Autodesk Inventor part; units mm, degrees
ref_plane "YZ Plane" through (0, 0, 0) normal (1, 0, 0) x (0, 1, 0)
ref_plane "XZ Plane" through (0, 0, 0) normal (0, 1, 0) x (-1, 0, 0)
ref_plane "XY Plane" through (0, 0, 0) normal (0, 0, 1) x (1, 0, 0)
sketch "Sketch1" plane through (0, 0, 0) normal (0, 1, 0) x (-1, 0, 0)
  circle A0 centre (0, 0) radius 13
  line L0 (-11.5, 0) -> (-9.303695, 6.75953) construction
  line L1 (-9.303695, 6.75953) -> (-3.553695, 10.93715) construction
  line L2 (-3.553695, 10.93715) -> (3.553695, 10.93715) construction
  line L3 (3.553695, 10.93715) -> (9.303695, 6.75953) construction
  line L4 (9.303695, 6.75953) -> (11.5, 0) construction
  line L5 (11.5, 0) -> (9.303695, -6.75953) construction
  line L6 (9.303695, -6.75953) -> (3.553695, -10.93715) construction
  line L7 (3.553695, -10.93715) -> (-3.553695, -10.93715) construction
  line L8 (-3.553695, -10.93715) -> (-9.303695, -6.75953) construction
  line L9 (-9.303695, -6.75953) -> (-11.5, 0) construction
  circle A1 centre (-6, 0) radius 3 construction
  circle A2 centre (6, 0) radius 3 construction
  line L10 (13, 0) -> (10.517221, -7.641208) construction
  line L11 (10.517221, -7.641208) -> (4.017221, -12.363735) construction
  line L12 (4.017221, -12.363735) -> (-4.017221, -12.363735) construction
  line L13 (-4.017221, -12.363735) -> (-10.517221, -7.641208) construction
  line L14 (-10.517221, -7.641208) -> (-13, 0) construction
  line L15 (-13, 0) -> (-10.517221, 7.641208) construction
  line L16 (-10.517221, 7.641208) -> (-4.017221, 12.363735) construction
  line L17 (-4.017221, 12.363735) -> (4.017221, 12.363735) construction
  line L18 (4.017221, 12.363735) -> (10.517221, 7.641208) construction
  line L19 (10.517221, 7.641208) -> (13, 0) construction
  dimension "d0" = 26
  dimension "d10" = 6
  dimension "d11" = 6
ref_plane "Work Plane1" through (0, -5, 0) normal (0, -1, 0) x (1, 0, 0)
sketch "Sketch2" plane through (0, -5, 0) normal (0, -1, 0) x (1, 0, 0)
  circle A0 centre (0, 0) radius 13 construction
  line L0 (-9.303695, 6.75953) -> (-11.5, 0)
  line L1 (-11.5, 0) -> (-9.303695, 6.75953)
  line L2 (-9.303695, 6.75953) -> (-3.553695, 10.93715)
  line L3 (-3.553695, 10.93715) -> (3.553695, 10.93715)
  line L4 (3.553695, 10.93715) -> (9.303695, 6.75953)
  line L5 (9.303695, 6.75953) -> (11.5, 0)
  line L6 (11.5, 0) -> (9.303695, -6.75953)
  line L7 (9.303695, -6.75953) -> (3.553695, -10.93715)
  line L8 (3.553695, -10.93715) -> (-3.553695, -10.93715)
  line L9 (-3.553695, -10.93715) -> (-9.303695, -6.75953)
  line L10 (-9.303695, -6.75953) -> (-11.5, 0)
sketch3d "3D Sketch1"
sketch "Sketch1 outline for Loft1" plane through (0, 0, 0) normal (0, 1, 0) x (-1, 0, 0)
  circle A0 centre (0, 0) radius 13
sketch "Sketch2 outline for Loft1" plane through (0, -5, 0) normal (0, -1, 0) x (1, 0, 0)
  line L0 (-11.5, 0) -> (-9.303695, 6.75953)
  line L1 (-9.303695, 6.75953) -> (-3.553695, 10.93715)
  line L2 (-3.553695, 10.93715) -> (3.553695, 10.93715)
  line L3 (3.553695, 10.93715) -> (9.303695, 6.75953)
  line L4 (9.303695, 6.75953) -> (11.5, 0)
  line L5 (11.5, 0) -> (9.303695, -6.75953)
  line L6 (9.303695, -6.75953) -> (3.553695, -10.93715)
  line L7 (3.553695, -10.93715) -> (-3.553695, -10.93715)
  line L8 (-3.553695, -10.93715) -> (-9.303695, -6.75953)
  line L9 (-9.303695, -6.75953) -> (-11.5, 0)
loft "Loft1" add profiles "Sketch1 outline for Loft1", "Sketch2 outline for Loft1"
sketch "Sketch3" plane through (0, 0, 0) normal (0, 1, 0) x (1, 0, 0)
  circle A0 centre (0, 0) radius 13
  line L0 (-11.5, 0) -> (-9.303695, 6.75953)
  line L1 (-9.303695, 6.75953) -> (-3.553695, 10.93715)
  line L2 (-3.553695, 10.93715) -> (3.553695, 10.93715)
  line L3 (3.553695, 10.93715) -> (9.303695, 6.75953)
  line L4 (9.303695, 6.75953) -> (11.5, 0)
  line L5 (11.5, 0) -> (9.303695, -6.75953)
  line L6 (9.303695, -6.75953) -> (3.553695, -10.93715)
  line L7 (3.553695, -10.93715) -> (-3.553695, -10.93715)
  line L8 (-3.553695, -10.93715) -> (-9.303695, -6.75953)
  line L9 (-9.303695, -6.75953) -> (-11.5, 0)
  circle A1 centre (0, 0) radius 13
  line L10 (-11.5, 0) -> (-9.303695, 6.75953)
  line L11 (-9.303695, 6.75953) -> (-3.553695, 10.93715)
  line L12 (-3.553695, 10.93715) -> (3.553695, 10.93715)
  line L13 (3.553695, 10.93715) -> (9.303695, 6.75953)
  line L14 (9.303695, 6.75953) -> (11.5, 0)
  line L15 (11.5, 0) -> (9.303695, -6.75953)
  line L16 (9.303695, -6.75953) -> (3.553695, -10.93715)
  line L17 (3.553695, -10.93715) -> (-3.553695, -10.93715)
  line L18 (-3.553695, -10.93715) -> (-9.303695, -6.75953)
  line L19 (-9.303695, -6.75953) -> (-11.5, 0)
  circle A2 centre (-6, 0) radius 3
  circle A3 centre (6, 0) radius 3
  dimension "d28" = 11.5
  dimension "d29" = 26
  dimension "d30" = 6
  dimension "d31" = 6
extrude "Extrusion4" cut sketch "Sketch3" against normal blind 5 contours A3
extrude "Extrusion5" cut sketch "Sketch3" against normal blind 5 contours A2
extrude "Extrusion6" add sketch "Sketch3" along normal blind 5 contours A0
properties part number "Probe P1.5"
Geometry: final body of the model. Coordinates: model frame, mm. A direction names the side the tool comes from. Round coordinates to 2 decimals unless told otherwise and drop trailing zeros. Order: outer loops, then holes, each group sorted by start corner. A loop starts at its lowest first (then second) coordinate and runs counter-clockwise, first axis right, second up. Notation, with made-up numbers: (-35, 60.5) -> (14, 60.5) arc R25 ccw to (14, 86.5) -> close; hole circle Ø9 at (49.5, 49.5). An arc over 180 degrees is marked (long way). Write each question's results on one line, items separated by ' | '.
Q1. Ray query, line 1 along X through (y, z) = (-3.35, 0) (3 decimals); line 2 along X through (y, z) = (-1.7, 0); line 3 along Y through (x, z) = (-6, 5). Return the intervals inside material, ascending.
Response values:
line 1: -11.995 to -9, -3 to 3, 9 to 11.995 | line 2: -12.49 to -9, -3 to 3, 9 to 12.49 | line 3: -5 to 0
Q2. Pull-direction query (Z, two-part tool) for faces 1 (the face through (-6.388, 2.465, 8.878)), 2 (the face through (-7, 5, 9)), 3 (the face through (-10.316, 2.465, -7.91)); classes: released by +Z, released by -Z, zero draft, split by the parting line, or undercut.
Response values:
face 1: undercut | face 2: zero draft | face 3: split by the parting line
Q3. Pin query (flat end, axial travel): pin 1 Ø1 at (x, y) = (10, 1.5) entering from +Z; pin 2 Ø1.5 at (x, y) = (-9, -3.5) entering from -Z; pin 3 Ø10 at (x, z) = (-0.5, 0) entering from +Y. Return the tip coordinate at first contact, or that it passes through.
Response values:
pin 1: z = 8.87 | pin 2: z = -8.34 | pin 3: y = 0
Q4. Section query A-A (y = 3.75). Output: boundary loops of the cut face in (x, z), and give its area (3 significant figures).
Response values:
outline: circle Ø26 at (0, 0); hole (-11.5, 0) -> (-9.3, -6.76) -> (-3.55, -10.94) -> (3.55, -10.94) -> (9.3, -6.76) -> (11.5, 0) -> (9.3, 6.76) -> (3.55, 10.94) -> (-3.55, 10.94) -> (-9.3, 6.76) -> close | area: 142 mm²
Q5. Section query B-B (z = -2.25). Count the separate pieces of the cut face and the enclosed holes in it, and give its area (3 significant figures).
Response values:
separate pieces: 3 | enclosed holes: 0 | area: 98.6 mm²
Q6. Access query for faces 4 (the face through (0, 2, -10.937)), 5 (the face through (8.77, -2.46, 1.15)). Directions: +Z, -Z, +X, -X, +Y, -Y. A direction counts if a zero-diameter tool reaches every point of the face in a straight line with its end or side. Return the directions, or none.
Response values:
face 4: +Y | face 5: +Y, -Y
